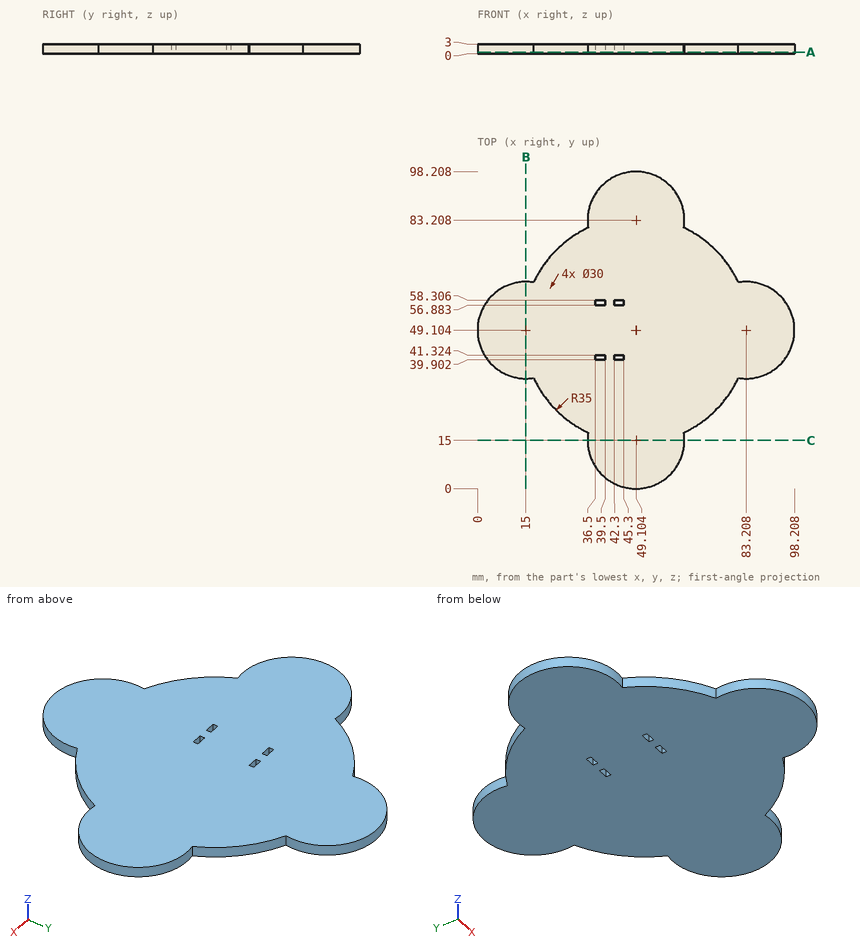
Verification items for this drawing (mm, ordinates from the low corner). Give positions to 0.01 mm unless a question says otherwise; leave off trailing zeros. Write each loop counter-clockwise with the first axis right and the second up, starting at its lowest first coordinate (ties: lowest second). Pieces come first, ordered by that corner, then holes. Notation, with made-up numbers: (87, -19) -> (98, -19) arc R26 ccw to (98, 1) -> close; hole circle Ø6 at (25.25, 59). An arc over 180 degrees is marked (long way). Write item = value, one per line.
Item 1: Sectioned sample at A-A on z = 0.45. Record the boundary of the cut face in (x, y) (1 decimal).
Output:
outline = (17.4, 34.3) arc R35 ccw to (34.3, 17.4) arc R15 ccw (long way) to (63.9, 17.4) arc R35 ccw to (80.8, 34.3) arc R15 ccw (long way) to (80.8, 63.9) arc R35 ccw to (63.9, 80.8) arc R15 ccw (long way) to (34.3, 80.8) arc R35 ccw to (17.4, 63.9) arc R15 ccw (long way) to start; hole (36.5, 39.9) -> (39.5, 39.9) -> (39.5, 41.3) -> (36.5, 41.3) -> close; hole (36.5, 56.9) -> (39.5, 56.9) -> (39.5, 58.3) -> (36.5, 58.3) -> close; hole (42.3, 39.9) -> (45.3, 39.9) -> (45.3, 41.3) -> (42.3, 41.3) -> close; hole (42.3, 56.9) -> (45.3, 56.9) -> (45.3, 58.3) -> (42.3, 58.3) -> close
Item 2: Sectioned sample at B-B on x = 15. Record the boundary of the cut face in (y, z).
Output:
outline = (34.1, 0) -> (64.1, 0) -> (64.1, 3) -> (34.1, 3) -> close
Item 3: Scan lines: probe 1 along Y at (x, z) = (38.5, 1.55) (1 decimal); probe 2 along Y at (x, z) = (44.5, 0.2) (1 decimal); probe 3 along Y at (x, z) = (77, 1.35) (1 decimal). Record each from-to range of solid material in increasing order. Write a range as from..to.
Output:
probe_1 = 4.4..39.9, 41.3..56.9, 58.3..93.8
probe_2 = 0.7..39.9, 41.3..56.9, 58.3..97.5
probe_3 = 28..70.2
Item 4: Gauge pin test, flat ends, axial feed: pin 1 (1.5 mm diameter, centred on x = 37.5, z = 1.5, fed in from +Y); pin 2 (0.9 mm diameter, centred on x = 43, z = 2, fed in from -Y); pin 3 (0.7 mm diameter, centred on y = 40.5, z = 1, fed in from -X) (1 decimal); pin 4 (12 mm diameter, centred on x = 81.5, y = 40, fed in from -Z). Record the tip position at first contact, or that the pin passes through.
Output:
pin_1 = 93.56
pin_2 = 1.11
pin_3 = 2.5
pin_4 = 0
